Design review of the part built by this model. Coordinates are the model's own, in mm. Face numbers are marked on the shaded views. A direction names the side the tool comes from. Give positions to 0.01 mm unless a question says otherwise; leave off trailing zeros. Write each loop counter-clockwise with the first axis right and the second up, starting at its lowest first coordinate (ties: lowest second). Pieces come first, ordered by that corner, then holes. Notation, with made-up numbers: (21, -3) -> (47, -3) arc R13 cw to (47, 9) -> close; hole circle Ø7 at (46.5, 84.5). An arc over 180 degrees is marked (long way). Put each result on its own line as item: value. Start each with the question number.
from build123d import *

# Parameters (mm, degrees)
SKETCH_1_W          = 20
SKETCH_1_H          = 20
EXTRUDE_1_DEPTH     = 30
SKETCH_2_W          = 20
SKETCH_2_H          = 20
EXTRUDE_2_DEPTH     = 40
SKETCH_6_W          = 20
SKETCH_6_H          = 20
EXTRUDE_3_DEPTH     = 30
SKETCH_7_W          = 20
SKETCH_7_H          = 20
EXTRUDE_4_DEPTH     = 60
SKETCH_8_R          = 3
CUT_EXTRUDE_1_DEPTH = 60


with BuildPart() as part:
    # 草图1 → 凸台-拉伸1 (new body)
    with BuildSketch(Plane(origin=(0, 0, 0), x_dir=(1, 0, 0), z_dir=(0, 1, 0))):
        Rectangle(SKETCH_1_W, SKETCH_1_H)
    extrude(amount=EXTRUDE_1_DEPTH)

    # 草图2 → 凸台-拉伸2 (add)
    with BuildSketch(Plane(origin=(10, 0, 0), x_dir=(0, 0, -1), z_dir=(1, 0, 0))):
        with Locations((0, 20)):
            Rectangle(SKETCH_2_W, SKETCH_2_H)
    extrude(amount=EXTRUDE_2_DEPTH)

    # 草图6 → 凸台-拉伸3 (add)
    with BuildSketch(Plane.XZ.offset(-10)):
        with Locations((40, 0)):
            Rectangle(SKETCH_6_W, SKETCH_6_H)
    extrude(amount=EXTRUDE_3_DEPTH)

    # 草图7 → 凸台-拉伸4 (add)
    with BuildSketch(Plane(origin=(0, 0, -10), x_dir=(-1, 0, 0), z_dir=(0, 0, -1))):
        with Locations((-40, -10)):
            Rectangle(SKETCH_7_W, SKETCH_7_H)
    extrude(amount=EXTRUDE_4_DEPTH)

    # 草图8 → 切除-拉伸1 (cut)
    with BuildSketch(Plane(origin=(0, 0, 0), x_dir=(-1, 0, 0), z_dir=(0, -1, 0))):
        with Locations(Location((0, 0, 0), (0, 0, 90))):
            Circle(SKETCH_8_R)
    extrude(amount=-CUT_EXTRUDE_1_DEPTH, mode=Mode.SUBTRACT)


solid = part.part
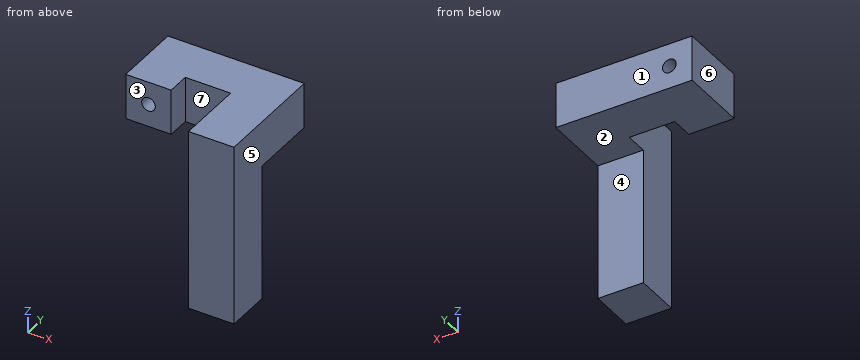
Q1. Take a section at C-C on z = 0. Give the boundary of the cut face in (x, y), then the cut area to 3 significant figures.
Q2. To check wall thickness, follow probe 1 along X at (y, z) = (17, 0); probe 2 along X at (y, z) = (8, 0); probe 3 along Z at (x, y) = (8, 5.5). State the ranges of each line that lie inside material, in increasing order. Write a range as from..to.
Q3. Take a section at B-B on x = 0. Give the boundary of the cut face in (y, z).
Q4. Machinability: for the marked faces 1, 2 and 3, which of the approach directions +Z, -Z, +X, -X, +Y, -Y give a long, thin tool a straight path to every point of the face, cutting with its end or side? Answer none if there is none.
Q5. Take a section at A-A on y = 1. Give the boundary of the cut face in (x, z).
Q6. Mouldability with a two-part tool opening along X and no side actions: class the marked faces 4, 5, 6 and 7 as +X half, -X half, draft (parallel to the pull), parting line (faces both ways), or undercut.
Q7. For pin 1 (6 mm diameter, centred on x = -3.5, z = -2.5, fed in from -Y); pin 2 (15 mm diameter, centred on x = 30, y = 21.5, fed in from -Z); pin 3 (10 mm diameter, centred on x = 19.5, z = 1.5, fed in from -Y), all flat-tipped, find the tip position at first contact; note any pin that passes through.
Q8. Take a section at D-D on z = -9. Give the boundary of the cut face in (x, y).
Result:
1. outline: (-10, 0) -> (-3, 0) -> (-3, 30) -> (-10, 30) -> close; (3, 0) -> (10, 0) -> (10, 10) -> (30, 10) -> (30, -20) -> (50, -20) -> (50, 30) -> (3, 30) -> close
1. area: 1,820 mm^2
2. probe 1: x = -10..-3, 3..50
2. probe 2: x = -10..-3, 3..10, 30..50
2. probe 3: z = -10..10
3. outline: (0, -10) -> (30, -10) -> (30, -3) -> (0, -3) -> close; (0, 3) -> (30, 3) -> (30, 10) -> (0, 10) -> close
4. face 1: +Z, -Z, +X, -X, +Y
4. face 2: -Z, +X, -X, +Y
4. face 3: +Z, -Z, -X, -Y
5. outline: (-10, -10) -> (10, -10) -> (10, 10) -> (-10, 10) -> close; (30, -10) -> (50, -10) -> (50, 10) -> (30, 10) -> close; hole circle Ø6 at (0, 0)
6. face 4: draft
6. face 5: +X half
6. face 6: -X half
6. face 7: undercut
7. pin 1: stops at y = 0
7. pin 2: stops at z = -10
7. pin 3: stops at y = 10
8. outline: (-10, 0) -> (10, 0) -> (10, 10) -> (30, 10) -> (30, -20) -> (50, -20) -> (50, 30) -> (-10, 30) -> close
